from build123d import *

# Parameters (mm, degrees)
F0_W         = 2.5711264648
F0_H         = 5
F1_DEPTH     = 3
F0_W_2       = 56.75
F0_H_2       = 56.75
F2_DEPTH     = 1
F3_R         = 1
F6_DEPTH     = 3
F7_T1_DEPTH  = 12.5
F7_T3_DEPTH  = 7.5711264648
F7_T5_DEPTH  = 3.5
F7_T8_ANGLE  = 90
F7_T10_ANGLE = 90


# Not quite as in the source:
# - a fillet or chamfer that OpenCascade refuses, or shapes differently, is made with other operations: its cross-section is extruded or revolved along the edge and cut away or added
# - a feature names something its author has since deleted; it is built from what else it names


with BuildPart() as f1:
    # F0 (on Top) → F1 (new body)
    with BuildSketch(Plane.XY):
        Polygon((-63.25, -34.2033516131), (-63.25, 26.5466483869), (-20, 26.5466483869), (-20, 31.5466483869), (-34.125, 31.5466483869), (-68.25, 31.5466483869), (-68.25, -36.7033516131), (0, -36.7033516131), (0, 31.5466483869), (-17.4288735352, 31.5466483869), (-17.4288735352, 26.5466483869), (-2.5, 26.5466483869), (-2.5, -34.2033516131), align=None)
        with Locations((-18.7144367676, 29.0466483869)):
            Rectangle(F0_W, F0_H)
    extrude(amount=F1_DEPTH)

    # F0 (on Top) → F2 (join)
    with BuildSketch(Plane.XY):
        Polygon((-20, 26.5466483869), (-63.25, 26.5466483869), (-63.25, -34.2033516131), (-2.5, -34.2033516131), (-2.5, 26.5466483869), (-17.4288735352, 26.5466483869), align=None)
        with Locations((-32.875, -3.8283516131)):
            Rectangle(F0_W_2, F0_H_2, mode=Mode.SUBTRACT)
    extrude(amount=F2_DEPTH)

    # F3
    f3_edges = [f1.edges().sort_by_distance(p)[0] for p in [
        (-32.875, 26.546648, 3),
        (-63.25, -3.828352, 3),
        (-32.875, -34.203352, 3),
        (-2.5, -3.828352, 3),
        (-34.125, 31.546648, 3),
        (-68.25, -2.578352, 3),
    ]]
    fillet(f3_edges, radius=F3_R)

    # F4: F1 across plane


with BuildPart() as f1_1:
    add(f1.part)
    add(f1.part.mirror(Plane.YZ))

    # F5: F1 across face


with BuildPart() as f1_2:
    add(f1_1.part)
    add(f1_1.part.mirror(Plane(origin=(0, -36.7033516131, 1.4986605371), x_dir=(1, 0, 0), z_dir=(0, -1, 0))))

    # F0 (on Top) → F6 (join)
    with BuildSketch(Plane.XY):
        with BuildLine():
            ThreePointArc((-10, 41.5466483869), (-17.0710678119, 38.6177161988), (-20, 31.5466483869))
            Line((-20, 31.5466483869), (-17.4288735352, 31.5466483869))
            ThreePointArc((-17.4288735352, 31.5466483869), (-15.2530068533, 36.7996552402), (-10, 38.9755219221))
            Line((-10, 38.9755219221), (0, 38.9755219221))
            Line((0, 38.9755219221), (0, 41.5466483869))
            Line((0, 41.5466483869), (-10, 41.5466483869))
        make_face()
        with Locations((-18.7144367676, 29.0466483869)):
            Rectangle(F0_W, F0_H)
    extrude(amount=F6_DEPTH)

    # F7: fillet of radius 1 on 4 edges, made by hand

    # F7_s2 → F7_t1 (cut)
    with BuildSketch(Plane.YZ.offset(-10)):
        with BuildLine():
            ThreePointArc((39.9755219221, 3), (39.2684151409, 2.7071067812), (38.9755219221, 2))
            Line((38.9755219221, 2), (38.9755219221, 3))
            Line((38.9755219221, 3), (39.9755219221, 3))
        make_face()
        with BuildLine():
            ThreePointArc((40.5466483869, 3), (41.2537551681, 2.7071067812), (41.5466483869, 2))
            Line((41.5466483869, 2), (41.5466483869, 3))
            Line((41.5466483869, 3), (40.5466483869, 3))
        make_face()
    extrude(amount=F7_T1_DEPTH, mode=Mode.SUBTRACT)

    # F7_s4 → F7_t3 (cut)
    with BuildSketch(Plane.YZ.offset(-22.5)):
        with BuildLine():
            ThreePointArc((27.5466483869, 3), (26.8395416057, 2.7071067812), (26.5466483869, 2))
            Line((26.5466483869, 2), (26.5466483869, 3))
            Line((26.5466483869, 3), (27.5466483869, 3))
        make_face()
    extrude(amount=F7_T3_DEPTH, mode=Mode.SUBTRACT)

    # F7_s6 → F7_t5 (cut)
    with BuildSketch(Plane.XZ.offset(-31.5466483869)):
        with BuildLine():
            ThreePointArc((-19, 3), (-19.7071067812, 2.7071067812), (-20, 2))
            Line((-20, 2), (-20, 3))
            Line((-20, 3), (-19, 3))
        make_face()
        with BuildLine():
            ThreePointArc((-18.4288735352, 3), (-17.721766754, 2.7071067812), (-17.4288735352, 2))
            Line((-17.4288735352, 2), (-17.4288735352, 3))
            Line((-17.4288735352, 3), (-18.4288735352, 3))
        make_face()
    extrude(amount=F7_T5_DEPTH, mode=Mode.SUBTRACT)

    # F7_s7 → F7_t8 (revolve, cut)
    with BuildSketch(Plane.XZ.offset(-31.5466483869)):
        with BuildLine():
            ThreePointArc((-18.4288735352, 3), (-17.721766754, 2.7071067812), (-17.4288735352, 2))
            Line((-17.4288735352, 2), (-17.4288735352, 3))
            Line((-17.4288735352, 3), (-18.4288735352, 3))
        make_face()
    revolve(axis=Axis((-10, 31.5466483869, 3), (0, 0, -1)), revolution_arc=F7_T8_ANGLE, mode=Mode.SUBTRACT)

    # F7_s9 → F7_t10 (revolve, cut)
    with BuildSketch(Plane.YZ.offset(-10)):
        with BuildLine():
            ThreePointArc((40.5466483869, 3), (41.2537551681, 2.7071067812), (41.5466483869, 2))
            Line((41.5466483869, 2), (41.5466483869, 3))
            Line((41.5466483869, 3), (40.5466483869, 3))
        make_face()
    revolve(axis=Axis((-10, 31.5466483869, 3), (0, 0, 1)), revolution_arc=F7_T10_ANGLE, mode=Mode.SUBTRACT)

    # F8: F1 across plane


with BuildPart() as f1_3:
    add(f1_2.part)
    add(f1_2.part.mirror(Plane.YZ))


solid = f1_3.part
Input: part model. Units: mm. Frame: model coordinates. A direction names the side the tool comes from. Coordinates: 2 decimals unless noted, no trailing zeros. Order: outer loops, then holes, each group sorted by start corner. A loop starts at its lowest first (then second) coordinate and runs counter-clockwise, first axis right, second up. Notation, with made-up numbers: M -11,37.25 L 40,37.25 A8 cw 40,41.25 Z; hole C 62.5,0.25 d8. An arc over 180 degrees is marked long. Answer in a Markdown table with one row per item.
(1) Material intervals for line 1 (X direction, y = -21, z = 1.4); line 2 (Y direction, x = -39, z = 1.3); line 3 (Y direction, x = -45, z = 0.25), sorted ascending. Write a range as [from, to].
Numbers:
| item | result |
|---|---|
| line 1 | x = [-68.25, -63.25], [-2.5, 2.5], [63.25, 68.25] |
| line 2 | y = [-104.95, -99.95], [-39.2, -34.2], [26.55, 31.55] |
| line 3 | y = [-104.95, -97.95], [-41.2, -32.2], [24.55, 31.55] |
(2) Access query for faces 4 (the cylindrical face through (-16.99, 38.7, 0.99)), 5 (the cylindrical face through (-15.31, 36.74, 0.99)), 6 (the flat face through (-35, -33, 1)). Directions: +Z, -Z, +X, -X, +Y, -Y. A direction counts if a zero-diameter tool reaches every point of the face in a straight line with its end or side. Return the directions, or none.
Numbers:
| item | result |
|---|---|
| face 4 | +Z, -Z, -X, +Y |
| face 5 | +Z, -Z |
| face 6 | +Z |
(3) Contact query for flat-ended pins moving along their axis: pin 1 Ø0.8 at (x, z) = (-35.5, 1.5) entering from +Y; pin 2 Ø6 at (x, y) = (-39, -46) entering from -Z. Output: stop coordinate, or through.
Numbers:
| item | result |
|---|---|
| pin 1 | stops at y = 31.55 |
| pin 2 | passes through |
(4) Section query A-A, the plane y = -92.5. Output: boundary loops of the cut face in (x, z).
Numbers:
| item | result |
|---|---|
| outline | M -68.25,0 L -61.25,0 L -61.25,1 L -63.25,1 L -63.25,2 A1 ccw -64.25,3 L -67.25,3 A1 ccw -68.25,2 Z; M -4.5,0 L 4.5,0 L 4.5,1 L 2.5,1 L 2.5,2 A1 ccw 1.5,3 L -1.5,3 A1 ccw -2.5,2 L -2.5,1 L -4.5,1 Z; M 61.25,0 L 68.25,0 L 68.25,2 A1 ccw 67.25,3 L 64.25,3 A1 ccw 63.25,2 L 63.25,1 L 61.25,1 Z |
(5) Section query C-C, the plane x = -13.5. Give the number of separate pieces and of enclosed holes in the cut face, plus the area to 3 significant figures.
Numbers:
| item | result |
|---|---|
| separate pieces | 4 |
| enclosed holes | 0 |
| area | 59.7 mm^2 |
(6) Draft query along X for faces 1 (the cylindrical face through (16.99, 38.7, 0.99)), 2 (the flat face through (35, -33, 1)), 3 (the flat face through (0, -31, 0)). Return one class per face: pulls with the +X half, pulls with the -X half, needs draft (parallel to the pull), parting line crosses it, or undercut.
Numbers:
| item | result |
|---|---|
| face 1 | pulls with the +X half |
| face 2 | undercut |
| face 3 | needs draft |
(7) Section query B-B, the plane x = -37.5. Output: boundary loops of the cut face in (y, z), plus the area to 3 significant figures.
Numbers:
| item | result |
|---|---|
| outline | M -104.95,0 L -97.95,0 L -97.95,1 L -99.95,1 L -99.95,2 A1 ccw -100.95,3 L -103.95,3 A1 ccw -104.95,2 Z; M -41.2,0 L -32.2,0 L -32.2,1 L -34.2,1 L -34.2,2 A1 ccw -35.2,3 L -38.2,3 A1 ccw -39.2,2 L -39.2,1 L -41.2,1 Z; M 24.55,0 L 31.55,0 L 31.55,2 A1 ccw 30.55,3 L 27.55,3 A1 ccw 26.55,2 L 26.55,1 L 24.55,1 Z |
| area | 51.7 mm^2 |
